```python
from build123d import *

# Parameters (mm, degrees)
SKETCH1_W                  = 225
SKETCH1_H                  = 77.5
SKETCH1_R                  = 2
BOSS_EXTRUDE1_DEPTH        = 3
SKETCHED_START             = -27.618786464
SKETCHED_BEND1_OUTLINE_W   = 225
SKETCHED_BEND1_OUTLINE_H   = 3
SKETCHED_BEND1_DEPTH       = 62.248893571
SKETCHED_START_2           = 35.116407107
SKETCHED_BEND1_2_OUTLINE_W = 225
SKETCHED_BEND1_2_OUTLINE_H = 50.002212856
SKETCHED_BEND1_2_OUTLINE_R = 2
SKETCHED_BEND1_2_DEPTH     = 2.5137
SKETCHED_START_3           = 39.630107107
SKETCHED_BEND1_3_OUTLINE_W = 225
SKETCHED_BEND1_3_OUTLINE_H = 3
SKETCHED_BEND1_3_DEPTH     = 10.251106429
SKETCHED_START_4           = 34.630107107
SKETCHED_BEND1_4_OUTLINE_W = 225
SKETCHED_BEND1_4_OUTLINE_H = 3
SKETCHED_BEND1_4_DEPTH     = 0.28314
SKETCHED_BEND1_5_OUTLINE_W = 225
SKETCHED_BEND1_5_OUTLINE_H = 50.002212856
SKETCHED_BEND1_5_OUTLINE_R = 2
SKETCHED_BEND1_5_DEPTH     = 5
SKETCHED_START_5           = -66.5
SKETCHED_BEND1_6_DEPTH     = 225
SKETCHED_BEND1_7_DEPTH     = 225


with BuildPart() as part:
    # Sketch1 → Boss-Extrude1 (new body)
    with BuildSketch(Plane(origin=(0, 0, 0), x_dir=(1, 0, 0), z_dir=(0, 1, 0))):
        with Locations((46, -11.131213536)):
            Rectangle(SKETCH1_W, SKETCH1_H)
        with Locations(Location((38.5, 1.368786464, 0), (0, 0, 270))):
            Circle(SKETCH1_R, mode=Mode.SUBTRACT)
        with Locations(Location((38.5, -23.631213536, 0), (0, 0, 90))):
            Circle(SKETCH1_R, mode=Mode.SUBTRACT)
        with Locations(Location((51.5, 1.368786464, 0), (0, 0, 270))):
            Circle(SKETCH1_R, mode=Mode.SUBTRACT)
        with Locations(Location((51.5, -23.631213536, 0), (0, 0, 90))):
            Circle(SKETCH1_R, mode=Mode.SUBTRACT)
        with Locations(Location((64.5, 1.368786464, 0), (0, 0, 270))):
            Circle(SKETCH1_R, mode=Mode.SUBTRACT)
        with Locations(Location((64.5, -23.631213536, 0), (0, 0, 90))):
            Circle(SKETCH1_R, mode=Mode.SUBTRACT)
    extrude(amount=BOSS_EXTRUDE1_DEPTH)

    # Sketched Bend1: read off the stored shape, not the designer's step
    # Sketched Bend1 outline → Sketched Bend1 (cut)
    with BuildSketch(Plane.XY.offset(SKETCHED_START)):
        with Locations((46, 1.5)):
            Rectangle(SKETCHED_BEND1_OUTLINE_W, SKETCHED_BEND1_OUTLINE_H)
    extrude(amount=SKETCHED_BEND1_DEPTH, mode=Mode.SUBTRACT)

    # Sketched Bend1 2 outline → Sketched Bend1 2 (add)
    with BuildSketch(Plane.XY.offset(SKETCHED_START_2)):
        with Locations((46, 28.001106428)):
            Rectangle(SKETCHED_BEND1_2_OUTLINE_W, SKETCHED_BEND1_2_OUTLINE_H)
        with Locations((38.5, 15.501106428)):
            Circle(SKETCHED_BEND1_2_OUTLINE_R, mode=Mode.SUBTRACT)
        with Locations((51.5, 15.501106428)):
            Circle(SKETCHED_BEND1_2_OUTLINE_R, mode=Mode.SUBTRACT)
        with Locations((64.5, 15.501106428)):
            Circle(SKETCHED_BEND1_2_OUTLINE_R, mode=Mode.SUBTRACT)
        with Locations((38.5, 40.501106428)):
            Circle(SKETCHED_BEND1_2_OUTLINE_R, mode=Mode.SUBTRACT)
        with Locations((51.5, 40.501106428)):
            Circle(SKETCHED_BEND1_2_OUTLINE_R, mode=Mode.SUBTRACT)
        with Locations((64.5, 40.501106428)):
            Circle(SKETCHED_BEND1_2_OUTLINE_R, mode=Mode.SUBTRACT)
    extrude(amount=SKETCHED_BEND1_2_DEPTH)

    # Sketched Bend1 4 outline → Sketched Bend1 4 (cut)
    with BuildSketch(Plane.XY.offset(SKETCHED_START_4)):
        with Locations((46, 1.5)):
            Rectangle(SKETCHED_BEND1_4_OUTLINE_W, SKETCHED_BEND1_4_OUTLINE_H)
    extrude(amount=SKETCHED_BEND1_4_DEPTH, mode=Mode.SUBTRACT)



with BuildPart() as body_2:
    # Sketched Bend1 3 outline → Sketched Bend1 3 (new body)
    with BuildSketch(Plane.XY.offset(SKETCHED_START_3)):
        with Locations((46, 54.502212856)):
            Rectangle(SKETCHED_BEND1_3_OUTLINE_W, SKETCHED_BEND1_3_OUTLINE_H)
    extrude(amount=SKETCHED_BEND1_3_DEPTH)


with BuildPart() as part_1:
    add(part.part)

    add(body_2.part)  # Sketched Bend1 5 merges body 2
    # Sketched Bend1 5 outline → Sketched Bend1 5 (add)
    with BuildSketch(Plane.XY.offset(SKETCHED_START_4)):
        with Locations((46, 28.001106428)):
            Rectangle(SKETCHED_BEND1_5_OUTLINE_W, SKETCHED_BEND1_5_OUTLINE_H)
        with Locations((38.5, 15.501106428)):
            Circle(SKETCHED_BEND1_5_OUTLINE_R, mode=Mode.SUBTRACT)
        with Locations((51.5, 15.501106428)):
            Circle(SKETCHED_BEND1_5_OUTLINE_R, mode=Mode.SUBTRACT)
        with Locations((64.5, 15.501106428)):
            Circle(SKETCHED_BEND1_5_OUTLINE_R, mode=Mode.SUBTRACT)
        with Locations((38.5, 40.501106428)):
            Circle(SKETCHED_BEND1_5_OUTLINE_R, mode=Mode.SUBTRACT)
        with Locations((51.5, 40.501106428)):
            Circle(SKETCHED_BEND1_5_OUTLINE_R, mode=Mode.SUBTRACT)
        with Locations((64.5, 40.501106428)):
            Circle(SKETCHED_BEND1_5_OUTLINE_R, mode=Mode.SUBTRACT)
    extrude(amount=SKETCHED_BEND1_5_DEPTH)

    # Sketched Bend1 6 outline → Sketched Bend1 6 (cut)
    with BuildSketch(Plane.YZ.offset(SKETCHED_START_5)):
        with BuildLine():
            Line((3, 34.630107107), (5, 34.630107107))
            ThreePointArc((5, 34.630107107), (1.464466094, 36.094573201), (0, 39.630107107))
            Line((0, 39.630107107), (0, 34.913247107))
            Line((0, 34.913247107), (3, 34.913247107))
            Line((3, 34.913247107), (3, 34.630107107))
        make_face()
        with BuildLine():
            Line((53.002212856, 34.630107107), (53.002212856, 35.047531413))
            ThreePointArc((53.002212856, 35.047531413), (52.023761074, 34.735575543), (51.002212856, 34.630107107))
            Line((51.002212856, 34.630107107), (53.002212856, 34.630107107))
        make_face()
        with BuildLine():
            Line((5, 37.630107107), (51.002212856, 37.630107107))
            ThreePointArc((51.002212856, 37.630107107), (52.416426419, 38.215893545), (53.002212856, 39.630107107))
            Line((53.002212856, 39.630107107), (3, 39.630107107))
            ThreePointArc((3, 39.630107107), (3.585786438, 38.215893545), (5, 37.630107107))
        make_face()
    extrude(amount=SKETCHED_BEND1_6_DEPTH, mode=Mode.SUBTRACT)

    # Sketched Bend1 7 outline → Sketched Bend1 7 (add)
    with BuildSketch(Plane.YZ.offset(SKETCHED_START_5)):
        with BuildLine():
            Line((56.002212856, 39.630107107), (53.002212856, 39.630107107))
            Line((53.002212856, 39.630107107), (53.002212856, 35.047531413))
            ThreePointArc((53.002212856, 35.047531413), (55.185512988, 36.89149432), (56.002212856, 39.630107107))
        make_face()
    extrude(amount=SKETCHED_BEND1_7_DEPTH)


solid = part_1.part
```
Check sheet for the modelled part. Datum: model origin and axes. Units: mm. A direction names the side the tool comes from. Give positions to 0.01 mm unless a question says otherwise; leave off trailing zeros. Loops run counter-clockwise (first coordinate to the right, second up) from the corner with the lowest first, then second, coordinate; pieces in that order, holes last. Notation, with made-up numbers: M 20,73.25 L 34,73.25 A32 ccw 34,99.25 Z; hole C -35,55.5 d8. An arc over 180 degrees is marked long. Answer as CSV lines item,"result".
Item 1: Sectioned sample at C-C, the plane x = 96. Enter the section's corners in (y, z), then the cut area to 4 significant figures.
Reply:
outline,"M 0,39.63 A5 ccw 5,34.63 L 51,34.63 A5 ccw 56,39.63 L 56,49.88 L 53,49.88 L 53,39.63 A2 cw 51,37.63 L 5,37.63 A2 cw 3,39.63 L 3,49.88 L 0,49.88 Z"
area,"232.5 mm^2"
Item 2: Set-up check for faces 4 (the face through (51.24, 42.484, 36.109)), 5 (the face through (44, 28, 37.63)): record each of +Z, -Z, +X, -X, +Y, -Y from which the full face is reachable in a straight line by a thin tool's end or side.
Reply:
face 4,"+Z, -Z"
face 5,"+Z, +X, -X"
Item 3: Sectioned sample at A-A, the plane x = 64.5. Enter the section's corners in (y, z), then the cut area to 4 significant figures.
Reply:
outline,"M 0,39.63 A5 ccw 5,34.63 L 13.5,34.63 L 13.5,37.63 L 5,37.63 A2 cw 3,39.63 L 3,49.88 L 0,49.88 Z; M 17.5,34.63 L 38.5,34.63 L 38.5,37.63 L 17.5,37.63 Z; M 42.5,34.63 L 51,34.63 A5 ccw 56,39.63 L 56,49.88 L 53,49.88 L 53,39.63 A2 cw 51,37.63 L 42.5,37.63 Z"
area,"208.5 mm^2"
Item 4: Sectioned sample at B-B, the plane z = 46. Enter the section's corners in (x, y).
Reply:
outline,"M -66.5,0 L 158.5,0 L 158.5,3 L -66.5,3 Z; M -66.5,53 L 158.5,53 L 158.5,56 L -66.5,56 Z"
Item 5: Depth check by flat-ended pin: pin 1 Ø12 at (x, y) = (-33, 14.5) entering from +Z. Enter the tip coordinate at first touch or a pass-through.
Reply:
pin 1,"z = 37.63"
Item 6: Sectioned sample at D-D, the plane y = 34.5. Enter the section's corners in (x, z), then the cut area to 3 significant figures.
Reply:
outline,"M -66.5,34.63 L 158.5,34.63 L 158.5,37.63 L -66.5,37.63 Z"
area,"675 mm^2"
Item 7: Scan lines: L1, parallel to Y at x = 64.5, z = 36.4; L2, parallel to Y at x = 80, z = 44; L3, parallel to Y at x = 51.5, z = 36. Record each from-to range of solid material in increasing order.
Reply:
L1,"1.18 to 13.5, 17.5 to 38.5, 42.5 to 54.82"
L2,"0 to 3, 53 to 56"
L3,"1.56 to 13.5, 17.5 to 38.5, 42.5 to 54.44"
Item 8: Draft check along Y on faces 1 (the face through (64.066, 13.549, 36.109)), 2 (the face through (44, 28, 34.63)), 3 (the face through (44.42, 1.5, 36.06)). Enter one of: pulls with the +Y half, pulls with the -Y half, needs draft (parallel to the pull), parting line crosses it, or undercut.
Reply:
face 1,"undercut"
face 2,"needs draft"
face 3,"pulls with the -Y half"
